Read the model definition and answer for the solid it produces. Units are mm, in the model's axes. Face numbers are marked on the shaded views. Coordinates: 2 decimals unless noted, no trailing zeros. Loops run counter-clockwise (first coordinate to the right, second up) from the corner with the lowest first, then second, coordinate; pieces in that order, holes last.
Q1. Section A-A (y = -7) is taken. Give the vertices of the cut face in (x, z).
Q2. Section B-B (x = 0) is taken. Give the vertices of the cut face in (y, z).
Q3. Section C-C (z = 47) is taken. Give the vertices of the cut face in (x, y), then the cut area to 3 significant figures.
Q4. Flat-ended cylindrical pins translate along their axes: P1, Ø2, axis at x = 1.5, z = 16, coming from the -Y side; P2, Ø4, axis at x = -4, y = 7, coming from the +Z side; P3, Ø5, axis at y = 3.5, z = 23, coming from the +X side. Find the tip coordinate at first contact, or state that the pin passes through.
Q5. Straight lines are drawn through the part: line 1 (X direction, y = 0, z = 25); line 2 (Y direction, x = 0, z = 46); line 3 (Z direction, x = -9, y = 1.5). For each, find the intervals that lie inside material, in ascending order.
Q6. The mould has two halves that part along X. Classify the marked faces 1, 2 and 3: pulls with the +X half, pulls with the -X half, needs draft (parallel to the pull), parting line crosses it, or undercut.
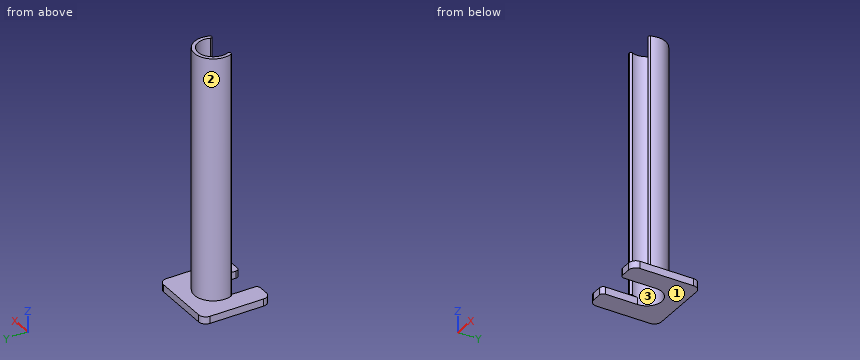
Autodesk Fusion 360 part; units mm, degrees
sketch "Skizze1" plane through (0, 0, 0) normal (0, 0, 1) x (1, 0, 0)
  line L0 (8, 9) -> (-8, 9)
  line L1 (-10, 7) -> (-10, -8)
  line L2 (10, -8) -> (10, 7)
  line L3 (-4.25, 0) -> (-4.25, -9)
  line L4 (4.25, 0) -> (4.25, -9)
  line L5 (-4.1679, -2.2229) -> (-4.1679, -2.2229)
  line L6 (4.1679, -2.2229) -> (4.1679, -2.2229)
  arc A0 (3.9397, -1.5942) -> (-3.9397, -1.5942) centre (0, 0) ccw
  arc A1 (4.8667, -1.9692) -> (-4.8667, -1.9692) centre (0, 0) ccw
  line L7 (-8, -10) -> (-5.25, -10)
  line L8 (5.25, -10) -> (8, -10)
  arc A2 (-8, 9) -> (-10, 7) centre (-8, 7) ccw
  arc A3 (10, 7) -> (8, 9) centre (8, 7) ccw
  arc A4 (-10, -8) -> (-8, -10) centre (-8, -8) ccw
  arc A5 (8, -10) -> (10, -8) centre (8, -8) ccw
  arc A6 (-5.25, -10) -> (-4.25, -9) centre (-5.25, -9) ccw
  arc A7 (4.25, -9) -> (5.25, -10) centre (5.25, -9) ccw
  arc A8 (-4.1679, -2.2229) -> (-3.9397, -1.5942) centre (-4.4032, -1.7817) ccw
  arc A9 (-4.8667, -1.9692) -> (-4.1679, -2.2229) centre (-4.4032, -1.7817) ccw
  arc A10 (3.9397, -1.5942) -> (4.1679, -2.2229) centre (4.4032, -1.7817) ccw
  arc A11 (4.1679, -2.2229) -> (4.8667, -1.9692) centre (4.4032, -1.7817) ccw
  dimension "d7" = 2
  dimension "d8" = 2
  dimension "d9" = 2
  dimension "d10" = 2
  dimension "d11" = 1
  dimension "d12" = 1
  dimension "d13" = 0.5
  dimension "d14" = 0.5
  dimension "d15" = 0.5
  dimension "d16" = 0.5
extrude "Extrusion4" add sketch "Skizze1" along normal blind 2 contours L0 L1 L2 L3 L4 A1 L7 L8 A2 A3 A4 A5 A6 A7 A9 A11 | L3 L4 A0 A1 A9 A11
extrude "Extrusion5" add sketch "Skizze1" along normal blind 70 and the other way blind -2 contours L4 A0 A10 A11 | L3 L4 A0 A1 A9 A11 | L3 A0 A8 A9
equation "d22 = Side2TaperAngle"
Numbers:
1. outline: (-10, 0) - (-4.25, 0) - (-4.25, 2) - (-10, 2) - close; (4.25, 0) - (10, 0) - (10, 2) - (4.25, 2) - close
2. outline: (4.25, 0) - (9, 0) - (9, 2) - (5.25, 2) - (5.25, 70) - (4.25, 70) - close
3. outline: (-4.87, -1.97) arc R0.5 ccw to (-4.17, -2.22) arc R0.5 ccw to (-3.94, -1.59) arc R4.25 cw (long way) to (3.94, -1.59) arc R0.5 ccw to (4.17, -2.22) arc R0.5 ccw to (4.87, -1.97) arc R5.25 ccw (long way) to start
3. area: 19.4 mm2
4. P1: stops at y = 3.44
4. P2: stops at z = 2
4. P3: stops at x = 5.15
5. line 1: x = -5.25 to -4.25, 4.25 to 5.25
5. line 2: y = 4.25 to 5.25
5. line 3: z = 0 to 2
6. face 1: needs draft
6. face 2: parting line crosses it
6. face 3: undercut
